from build123d import *

# Parameters (mm, degrees)
ESQUISSE1_W        = 900
ESQUISSE1_H        = 1860
ESQUISSE1_W_2      = 846
ESQUISSE1_H_2      = 1806
EXTRU_MINCE1_DEPTH = 60
ESQUISSE2_W        = 27
ESQUISSE2_H        = 1806
EXTRU_MINCE2_DEPTH = 60
ESQUISSE3_W        = 846
ESQUISSE3_H        = 27
EXTRU_MINCE3_DEPTH = 60


with BuildPart() as part:
    # Esquisse1 → Extru.-Mince1 (new body)
    with BuildSketch(Plane.XY):
        with Locations((450, 930)):
            Rectangle(ESQUISSE1_W, ESQUISSE1_H)
        with Locations((450, 930)):
            Rectangle(ESQUISSE1_W_2, ESQUISSE1_H_2, mode=Mode.SUBTRACT)
    extrude(amount=EXTRU_MINCE1_DEPTH)

    # Esquisse2 → Extru.-Mince2 (add)
    with BuildSketch(Plane.XY.offset(60)):
        with Locations((450, 930)):
            Rectangle(ESQUISSE2_W, ESQUISSE2_H)
    extrude(amount=-EXTRU_MINCE2_DEPTH)

    # Esquisse3 → Extru.-Mince3 (add)
    with BuildSketch(Plane.XY.offset(60)):
        with Locations((450, 930)):
            Rectangle(ESQUISSE3_W, ESQUISSE3_H)
    extrude(amount=-EXTRU_MINCE3_DEPTH)


solid = part.part
Geometry: final body of the model. Coordinates: model frame, mm. A direction names the side the tool comes from. Coordinates: 2 decimals unless noted, no trailing zeros. Loops run counter-clockwise (first coordinate to the right, second up) from the corner with the lowest first, then second, coordinate; pieces in that order, holes last. Notation, with made-up numbers: (-1, 48.25) - (56, 48.25) arc R29 ccw to (56, 68.25) - close; hole circle Ø8 at (24.25, 23). An arc over 180 degrees is marked (long way). Put each result on its own line as item: value. Start each with the question number.
Q1. Pin query (flat end, axial travel): pin 1 Ø5 at (y, z) = (325.5, 13) entering from -X. Return the tip coordinate at first contact, or that it passes through.
Q2. Cut plane B-B, the plane y = 1661. Return loops of the section in (x, z).
Q3. Cut plane A-A, the plane x = 775.5. Return loops of the section in (y, z).
Q4. Line query: line 1 (X direction, y = 1120, z = 17.5); line 2 (Y direction, x = 336, z = 26.5). Output: solid intervals per line, ascending.
Q5. Pull-direction query (Y, two-part tool) for faces 3 (the flat face through (444, 1860, 30)), 4 (the flat face through (900, 917, 30)), 5 (the flat face through (229, 1833, 30)); classes: released by +Y, released by -Y, zero draft, split by the parting line, or undercut.
Q6. Cut plane C-C, the plane z = 26.5. Return loops of the section in (x, y).
Q7. Set-up query: faces 1 (the flat face through (0, 917, 30)), 2 (the flat face through (436.5, 1382, 30)). Return all of +Z, -Z, +X, -X, +Y, -Y with unobstructed straight access to the full face (end or side cutting, diameter ignored); none if empty.
Filled sheet:
1. pin 1: x = 0
2. outline: (0, 0) - (27, 0) - (27, 60) - (0, 60) - close; (436.5, 0) - (463.5, 0) - (463.5, 60) - (436.5, 60) - close; (873, 0) - (900, 0) - (900, 60) - (873, 60) - close
3. outline: (0, 0) - (27, 0) - (27, 60) - (0, 60) - close; (916.5, 0) - (943.5, 0) - (943.5, 60) - (916.5, 60) - close; (1833, 0) - (1860, 0) - (1860, 60) - (1833, 60) - close
4. line 1: 0 to 27, 436.5 to 463.5, 873 to 900
4. line 2: 0 to 27, 916.5 to 943.5, 1833 to 1860
5. face 3: released by +Y
5. face 4: zero draft
5. face 5: undercut
6. outline: (0, 0) - (900, 0) - (900, 1860) - (0, 1860) - close; hole (27, 27) - (436.5, 27) - (436.5, 916.5) - (27, 916.5) - close; hole (27, 943.5) - (436.5, 943.5) - (436.5, 1833) - (27, 1833) - close; hole (463.5, 27) - (873, 27) - (873, 916.5) - (463.5, 916.5) - close; hole (463.5, 943.5) - (873, 943.5) - (873, 1833) - (463.5, 1833) - close
7. face 1: +Z, -Z, -X, +Y, -Y
7. face 2: +Z, -Z
